```python
from build123d import *

# Parameters (mm, degrees)
F1_DEPTH = 20
F2_R     = 2
F3_DEPTH = 25
F4_R     = 2
F5_R     = 2


with BuildPart() as f1:
    # F0 (on Front) → F1 (new body)
    with BuildSketch(Plane.XZ):
        Polygon((18, 0), (0, 0), (0, 16), (-2, 16), (-2, -14), (8, -14), (8, -4), (18, -4), align=None)
    extrude(amount=F1_DEPTH)

    # F2 (on face) → F3 (cut)
    with BuildSketch(Plane(origin=(0, 0, -4), x_dir=(1, 0, 0), z_dir=(0, 0, -1))):
        with Locations((13, 15)):
            Circle(F2_R)
        with Locations((13, 5)):
            Circle(F2_R)
    extrude(amount=-F3_DEPTH, mode=Mode.SUBTRACT)

    # F4
    f4_edges = [f1.edges().sort_by_distance(p)[0] for p in [
        (-2, -10, -14),
    ]]
    fillet(f4_edges, radius=F4_R)

    # F5
    f5_edges = [f1.edges().sort_by_distance(p)[0] for p in [
        (8, -10, -14),
    ]]
    fillet(f5_edges, radius=F5_R)


solid = f1.part
```
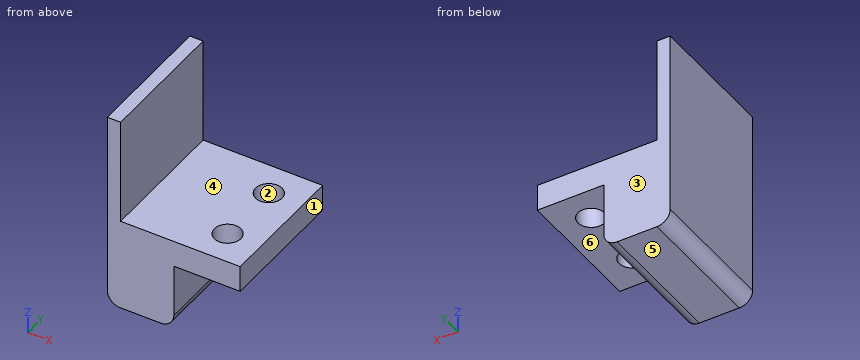
Can you work these out from the model? Positions are in its coordinate system, mm. Face numbers are marked on the shaded views. A direction names the side the tool comes from. Coordinates: 2 decimals unless noted, no trailing zeros. Order: outer loops, then holes, each group sorted by start corner. A loop starts at its lowest first (then second) coordinate and runs counter-clockwise, first axis right, second up. Notation, with made-up numbers: (76.25, 50) -> (116.25, 50) arc R13 cw to (116.25, 67) -> close; hole circle Ø3 at (26, 78.5). An arc over 180 degrees is marked (long way). Write each question's results on one line, items separated by ' | '.
Item 1: I want a section at B-B, the plane y = -15. Write out the boundary of the cut face in (x, z), then the cut area to 3 significant figures.
Results are:
outline: (-2, -12) arc R2 ccw to (0, -14) -> (6, -14) arc R2 ccw to (8, -12) -> (8, -4) -> (11, -4) -> (11, 0) -> (0, 0) -> (0, 16) -> (-2, 16) -> close; (15, -4) -> (18, -4) -> (18, 0) -> (15, 0) -> close | area: 194 mm²
Item 2: I want a section at A-A, the plane x = 13. Write out the boundary of the cut face in (y, z).
Results are:
outline: (-20, -4) -> (-17, -4) -> (-17, 0) -> (-20, 0) -> close; (-13, -4) -> (-7, -4) -> (-7, 0) -> (-13, 0) -> close; (-3, -4) -> (0, -4) -> (0, 0) -> (-3, 0) -> close
Item 3: I want a section at C-C, the plane z = -1.25. Write out the boundary of the cut face in (x, y).
Results are:
outline: (-2, -20) -> (18, -20) -> (18, 0) -> (-2, 0) -> close; hole circle Ø4 at (13, -15); hole circle Ø4 at (13, -5)
Item 4: If we mould it in two halves opening along Y, with no side actions, what happens to the marked faces 1, 2 and 3? For each: +Y half, -Y half, draft (parallel to the pull), parting line (faces both ways), or undercut.
Results are:
face 1: draft | face 2: undercut | face 3: +Y half
Item 5: I want a section at D-D, the plane z = -10.5. Write out the boundary of the cut face in (x, y).
Results are:
outline: (-2, -20) -> (8, -20) -> (8, 0) -> (-2, 0) -> close
Item 6: Which directions (+Z, -Z, +X, -X, +Y, -Y) give clear straight access to the entire face, cutting with the end or side of a thin tool? Please do the marked faces 4, 5 and 6.
Results are:
face 4: +Z, +X, +Y, -Y | face 5: -Z, +X, -X, +Y, -Y | face 6: -Z, +X, +Y, -Y
Item 7: I'm going to push flat-ended pins straight in: pin 1 Ø8 at (x, y) = (11, -11.5) entering from -Z; pin 2 Ø5 at (y, z) = (-7.5, 11) entering from +X; pin 3 Ø3 at (x, y) = (12.5, -16) entering from +Z. Where does each tip first touch, or does it pass through?
Results are:
pin 1: z = -13.73 | pin 2: x = 0 | pin 3: z = 0
Item 8: If I drill on line 1 along Y through (x, z) = (13, -1.75); line 2 along Z through (x, y) = (15, -14); line 3 along X through (y, z) = (-15, -1.1), over which ranges is the centre line in solid material (lowest first)?
Results are:
line 1: -20 to -17, -13 to -7, -3 to 0 | line 2: -4 to 0 | line 3: -2 to 11, 15 to 18
